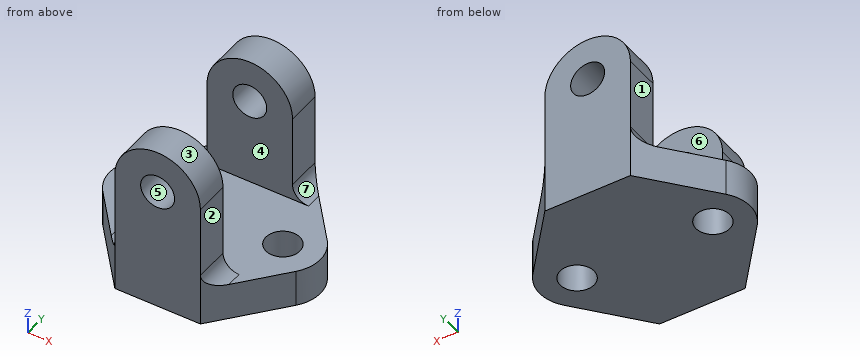
from build123d import *

# Parameters (mm, degrees)
SKETCH1_W                      = 41.4
SKETCH1_H                      = 33.02
SKETCH1_R                      = 3.175
BOSS_EXTRUDE1_DEPTH            = 9.46
SKETCH2_W                      = 41.4
SKETCH2_H                      = 6.51
BOSS_EXTRUDE2_DEPTH            = 53
CUT_EXTRUDE1_REACH             = 69.84
SKETCH4_R                      = 3.175
CUT_EXTRUDE1_DIRECTION_2_REACH = 69.84
CUT_EXTRUDE3_REACH             = 69.84
CUT_EXTRUDE3_DIRECTION_2_REACH = 69.84
CUT_EXTRUDE4_DEPTH             = 9.46
BOSS_EXTRUDE3_DEPTH            = 9.46
FILLET3_R                      = 3
CUT_EXTRUDE5_DEPTH             = 2.54


with BuildPart() as part:
    # Sketch1 → Boss-Extrude1 (new body)
    with BuildSketch(Plane.XY):
        Rectangle(SKETCH1_W, SKETCH1_H)
        with Locations((12.7, 0)):
            Circle(SKETCH1_R, mode=Mode.SUBTRACT)
        with Locations((-12.7, 0)):
            Circle(SKETCH1_R, mode=Mode.SUBTRACT)
    extrude(amount=BOSS_EXTRUDE1_DEPTH)

    # Sketch2 → Boss-Extrude2 (add)
    with BuildSketch(Plane.XY.offset(9.46)):
        with Locations((0, 13.255)):
            Rectangle(SKETCH2_W, SKETCH2_H)
        with Locations((0, -13.255)):
            Rectangle(SKETCH2_W, SKETCH2_H)
    extrude(amount=BOSS_EXTRUDE2_DEPTH)

    # Cut-Extrude1: up to this face of the body (flat: up to its plane)
    cut_extrude1_end = Plane(part.part.faces().sort_by_distance((0, -16.51, 31.23))[0])
    # Sketch4 → Cut-Extrude1 (cut, up to the picked face)
    with BuildSketch(Plane(origin=(0, 0, 0), x_dir=(1, 0, 0), z_dir=(0, 1, 0)), mode=Mode.PRIVATE) as cut_extrude1_sk1:
        with Locations(Location((0, -25.8481308, 0), (0, 0, 270))):
            Circle(SKETCH4_R)
    cut_extrude1_tool1 = split(extrude(cut_extrude1_sk1.sketch, amount=-CUT_EXTRUDE1_REACH, mode=Mode.PRIVATE), bisect_by=cut_extrude1_end, keep=Keep.BOTH, mode=Mode.PRIVATE)
    add(cut_extrude1_tool1.solids().sort_by(Axis((0, 0, 25.848131), (0, -1, 0)))[0], mode=Mode.SUBTRACT)

    # Cut-Extrude1 direction 2: up to this face of the body (flat: up to its plane)
    cut_extrude1_direction_2_end = Plane(part.part.faces().sort_by_distance((0, 16.51, 31.23))[0])
    # Sketch4 → Cut-Extrude1 direction 2 (cut, up to the picked face)
    with BuildSketch(Plane(origin=(0, 0, 0), x_dir=(1, 0, 0), z_dir=(0, 1, 0)), mode=Mode.PRIVATE) as cut_extrude1_direction_2_sk1:
        with Locations(Location((0, -25.8481308, 0), (0, 0, 270))):
            Circle(SKETCH4_R)
    cut_extrude1_direction_2_tool1 = split(extrude(cut_extrude1_direction_2_sk1.sketch, amount=CUT_EXTRUDE1_DIRECTION_2_REACH, mode=Mode.PRIVATE), bisect_by=cut_extrude1_direction_2_end, keep=Keep.BOTH, mode=Mode.PRIVATE)
    add(cut_extrude1_direction_2_tool1.solids().sort_by(Axis((0, 0, 25.848131), (0, 1, 0)))[0], mode=Mode.SUBTRACT)

    # Cut-Extrude3: up to this face of the body (flat: up to its plane)
    cut_extrude3_end = Plane(part.part.faces().sort_by_distance((0, -16.51, 31.296729805))[0])
    # Sketch6 → Cut-Extrude3 (cut, up to the picked face)
    with BuildSketch(Plane(origin=(0, 0, 0), x_dir=(1, 0, 0), z_dir=(0, 1, 0)), mode=Mode.PRIVATE) as cut_extrude3_sk1:
        with BuildLine():
            Line((-8, -25.8481308), (-8, -17.46))
            Line((-8, -17.46), (-8, -9.46))
            Line((-8, -9.46), (-16, -9.46))
            Line((-16, -9.46), (-20.7, -9.46))
            Line((-20.7, -9.46), (-20.7, -62.46))
            Line((-20.7, -62.46), (20.7, -62.46))
            Line((20.7, -62.46), (20.7, -9.46))
            Line((20.7, -9.46), (16, -9.46))
            Line((16, -9.46), (8, -9.46))
            Line((8, -9.46), (8, -17.46))
            Line((8, -17.46), (8, -25.8481308))
            ThreePointArc((8, -25.8481308), (0, -33.8481308), (-8, -25.8481308))
        make_face()
    cut_extrude3_tool1 = split(extrude(cut_extrude3_sk1.sketch, amount=-CUT_EXTRUDE3_REACH, mode=Mode.PRIVATE), bisect_by=cut_extrude3_end, keep=Keep.BOTH, mode=Mode.PRIVATE)
    add(cut_extrude3_tool1.solids().sort_by(Axis((0, 0, 38.949542), (0, -1, 0)))[0], mode=Mode.SUBTRACT)

    # Cut-Extrude3 direction 2: up to this face of the body (flat: up to its plane)
    cut_extrude3_direction_2_end = Plane(part.part.faces().sort_by_distance((0, 16.51, 31.296729805))[0])
    # Sketch6 → Cut-Extrude3 direction 2 (cut, up to the picked face)
    with BuildSketch(Plane(origin=(0, 0, 0), x_dir=(1, 0, 0), z_dir=(0, 1, 0)), mode=Mode.PRIVATE) as cut_extrude3_direction_2_sk1:
        with BuildLine():
            Line((-8, -25.8481308), (-8, -17.46))
            Line((-8, -17.46), (-8, -9.46))
            Line((-8, -9.46), (-16, -9.46))
            Line((-16, -9.46), (-20.7, -9.46))
            Line((-20.7, -9.46), (-20.7, -62.46))
            Line((-20.7, -62.46), (20.7, -62.46))
            Line((20.7, -62.46), (20.7, -9.46))
            Line((20.7, -9.46), (16, -9.46))
            Line((16, -9.46), (8, -9.46))
            Line((8, -9.46), (8, -17.46))
            Line((8, -17.46), (8, -25.8481308))
            ThreePointArc((8, -25.8481308), (0, -33.8481308), (-8, -25.8481308))
        make_face()
    cut_extrude3_direction_2_tool1 = split(extrude(cut_extrude3_direction_2_sk1.sketch, amount=CUT_EXTRUDE3_DIRECTION_2_REACH, mode=Mode.PRIVATE), bisect_by=cut_extrude3_direction_2_end, keep=Keep.BOTH, mode=Mode.PRIVATE)
    add(cut_extrude3_direction_2_tool1.solids().sort_by(Axis((0, 0, 38.949542), (0, 1, 0)))[0], mode=Mode.SUBTRACT)

    # Sketch7 → Cut-Extrude4 (cut)
    with BuildSketch(Plane.XY):
        with BuildLine():
            ThreePointArc((-12.7, -7), (-19.7, 0), (-12.7, 7))
            Line((-12.7, 7), (-8, 7))
            Line((-8, 7), (-8, 16.51))
            Line((-8, 16.51), (-20.7, 16.51))
            Line((-20.7, 16.51), (-20.7, -16.51))
            Line((-20.7, -16.51), (-8, -16.51))
            Line((-8, -16.51), (-8, -7))
            Line((-8, -7), (-12.7, -7))
        make_face()
        with BuildLine():
            Line((8, 16.51), (8, 7))
            Line((8, 7), (12.7, 7))
            ThreePointArc((12.7, 7), (19.7, 0), (12.7, -7))
            Line((12.7, -7), (8, -7))
            Line((8, -7), (8, -16.51))
            Line((8, -16.51), (20.7, -16.51))
            Line((20.7, -16.51), (20.7, 16.51))
            Line((20.7, 16.51), (8, 16.51))
        make_face()
    extrude(amount=CUT_EXTRUDE4_DEPTH, mode=Mode.SUBTRACT)

    # Sketch8 → Boss-Extrude3 (add)
    with BuildSketch(Plane.XY):
        with BuildLine():
            Line((8, -16.51), (18.065759147, -4.495400847))
            ThreePointArc((18.065759147, -4.495400847), (15.660759537, -6.343020019), (12.7, -7))
            Line((12.7, -7), (8, -7))
            Line((8, -7), (8, -16.51))
        make_face()
        with BuildLine():
            ThreePointArc((-18.065759147, -4.495400847), (-15.660759537, -6.343020019), (-12.7, -7))
            Line((-12.7, -7), (-8, -7))
            Line((-8, -7), (-8, -16.51))
            Line((-8, -16.51), (-18.065759147, -4.495400847))
        make_face()
        with BuildLine():
            Line((8, 16.51), (18.065759147, 4.495400847))
            ThreePointArc((18.065759147, 4.495400847), (15.660759537, 6.343020019), (12.7, 7))
            Line((12.7, 7), (8, 7))
            Line((8, 7), (8, 16.51))
        make_face()
        with BuildLine():
            Line((-8, 16.51), (-18.065759147, 4.495400847))
            ThreePointArc((-18.065759147, 4.495400847), (-15.660759537, 6.343020019), (-12.7, 7))
            Line((-12.7, 7), (-8, 7))
            Line((-8, 7), (-8, 16.51))
        make_face()
    extrude(amount=BOSS_EXTRUDE3_DEPTH)

    # Fillet3
    fillet3_edges = [part.edges().sort_by_distance(p)[0] for p in [
        (8, -13.255, 9.46),
        (-8, -13.255, 9.46),
        (8, 13.255, 9.46),
        (-8, 13.255, 9.46),
    ]]
    fillet(fillet3_edges, radius=FILLET3_R)

    # Sketch10 → Cut-Extrude5 (cut)
    with BuildSketch(Plane.XY):
        with BuildLine():
            Line((-8, 16.51), (-18.065759147, 4.495400847))
            ThreePointArc((-18.065759147, 4.495400847), (-19.7, 0), (-18.065759147, -4.495400847))
            Line((-18.065759147, -4.495400847), (-8, -16.51))
            Line((-8, -16.51), (8, -16.51))
            Line((8, -16.51), (18.065759147, -4.495400847))
            ThreePointArc((18.065759147, -4.495400847), (19.7, 0), (18.065759147, 4.495400847))
            Line((18.065759147, 4.495400847), (8, 16.51))
            Line((8, 16.51), (-8, 16.51))
        make_face()
    extrude(amount=CUT_EXTRUDE5_DEPTH, mode=Mode.SUBTRACT)


solid = part.part
The listing builds one solid part. Answer for the finished solid, in the listing's coordinates (mm). Face numbers are marked on the shaded views. A direction names the side the tool comes from. Coordinates: 2 decimals unless noted, no trailing zeros. Loops run counter-clockwise (first coordinate to the right, second up) from the corner with the lowest first, then second, coordinate; pieces in that order, holes last. Notation, with made-up numbers: (14, 64.25) -> (58, 64.25) arc R22 cw to (58, 78.25) -> close; hole circle Ø1 at (41.25, 32.5). An arc over 180 degrees is marked (long way). Answer in a Markdown table with one row per item. Add a question column.
1. For the marked faces 1, 2, 3 and 4, determine the directions among +Z, -Z, +X, -X, +Y, -Y from which every point of the face is accessible in a straight line to the end or side of a thin tool.
2. The part is cut by section C-C, the plane y = 0. Write down the section's boundary in (x, z) (3 decimals), then the cut area to 3 significant figures.
3. The part is cut by section A-A, the plane x = 0. Write down the section's boundary in (y, z).
4. Determine the mould class of the marked faces 5, 6 and 7 for opening direction X: +X half, -X half, draft (parallel to the pull), parting line (faces both ways), or undercut.
5. Consider line 1 (X direction, y = 0, z = 8.25) (3 decimals); line 2 (Y direction, x = -4, z = 23); line 3 (Z direction, x = 0, y = 12.5). Determine where each line is inside the solid, lowest interval first. Write a range as [from, to].
6. The part is cut by section B-B, the plane z = 28. Write down the section's boundary in (x, y).
7. The part is cut by section D-D, the plane z = 18. Write down the section's boundary in (x, y), then the cut area to 3 significant figures.
8. Flat-ended cylindrical pins translate along their axes: P1, Ø2, axis at y = -14.5, z = 18.5, coming from the +X side; P2, Ø5.5, axis at x = 0, z = 25.85, coming from the +Y side; P3, Ø8, axis at x = -9, z = 29, coming from the +Y side; P4, Ø3.5, axis at y = -12, z = 22, coming from the -X side. Find the tip coordinate at first contact, or state that the pin passes through.
Answer below:
| question | item | result |
|---|---|---|
| 1 | face 1 | +Z, -X, +Y, -Y |
| 1 | face 2 | +Z, +X, +Y, -Y |
| 1 | face 3 | +Z, +Y, -Y |
| 1 | face 4 | +Z, +X, -X |
| 2 | outline | (-19.7, 2.54) -> (-15.875, 2.54) -> (-15.875, 9.46) -> (-19.7, 9.46) -> close; (-9.525, 2.54) -> (9.525, 2.54) -> (9.525, 9.46) -> (-9.525, 9.46) -> close; (15.875, 2.54) -> (19.7, 2.54) -> (19.7, 9.46) -> (15.875, 9.46) -> close |
| 2 | area | 185 mm2 |
| 3 | outline | (-16.51, 2.54) -> (16.51, 2.54) -> (16.51, 22.67) -> (10, 22.67) -> (10, 9.46) -> (-10, 9.46) -> (-10, 22.67) -> (-16.51, 22.67) -> close; (-16.51, 29.02) -> (-10, 29.02) -> (-10, 33.85) -> (-16.51, 33.85) -> close; (10, 29.02) -> (16.51, 29.02) -> (16.51, 33.85) -> (10, 33.85) -> close |
| 4 | face 5 | undercut |
| 4 | face 6 | draft |
| 4 | face 7 | +X half |
| 5 | line 1 | [-19.7, -15.875], [-9.525, 9.525], [15.875, 19.7] |
| 5 | line 2 | [-16.51, -10], [10, 16.51] |
| 5 | line 3 | [2.54, 22.67], [29.02, 33.85] |
| 6 | outline | (-7.71, -16.51) -> (-2.33, -16.51) -> (-2.33, -10) -> (-7.71, -10) -> close; (-7.71, 10) -> (-2.33, 10) -> (-2.33, 16.51) -> (-7.71, 16.51) -> close; (2.33, -16.51) -> (7.71, -16.51) -> (7.71, -10) -> (2.33, -10) -> close; (2.33, 10) -> (7.71, 10) -> (7.71, 16.51) -> (2.33, 16.51) -> close |
| 7 | outline | (-8, -16.51) -> (8, -16.51) -> (8, -10) -> (-8, -10) -> close; (-8, 10) -> (8, 10) -> (8, 16.51) -> (-8, 16.51) -> close |
| 7 | area | 208 mm2 |
| 8 | P1 | x = 8 |
| 8 | P2 | through |
| 8 | P3 | y = 16.51 |
| 8 | P4 | x = -8 |
